Verification items for the finished model (mm, model axes). Face numbers are marked on the shaded views. A direction names the side the tool comes from. Give positions to 0.01 mm unless a question says otherwise; leave off trailing zeros. Order: outer loops, then holes, each group sorted by start corner. A loop starts at its lowest first (then second) coordinate and runs counter-clockwise, first axis right, second up.
from build123d import *

# Parameters (mm, degrees)
SKETCH1_W           = 21.9456
SKETCH1_H           = 10.033
SKETCH1_H_2         = 6.5151
BOSS_EXTRUDE1_DEPTH = 18.288
SKETCH2_W           = 15.748
SKETCH2_H           = 13.0048
BOSS_EXTRUDE2_DEPTH = 2.0066
SKETCH3_R           = 1.4605
CUT_EXTRUDE1_DEPTH  = 29.260148325


with BuildPart() as part:
    # Sketch1 → Boss-Extrude1 (new body)
    with BuildSketch(Plane(origin=(0, 0, 0), x_dir=(1, 0, 0), z_dir=(0, 1, 0))):
        with BuildLine():
            Line((-13.1826, -5.0165), (-10.9728, -5.0165))
            Line((-10.9728, -5.0165), (-10.9728, 5.0165))
            Line((-10.9728, 5.0165), (-13.1826, 5.0165))
            ThreePointArc((-13.1826, 5.0165), (-18.1991, 0), (-13.1826, -5.0165))
        make_face()
        Rectangle(SKETCH1_W, SKETCH1_H)
        with Locations((0, -8.27405)):
            Rectangle(SKETCH1_W, SKETCH1_H_2)
        with BuildLine():
            Line((10.9728, 5.0165), (10.9728, -5.0165))
            Line((10.9728, -5.0165), (13.1826, -5.0165))
            ThreePointArc((13.1826, -5.0165), (18.1991, 0), (13.1826, 5.0165))
            Line((13.1826, 5.0165), (10.9728, 5.0165))
        make_face()
        with Locations((0, 8.27405)):
            Rectangle(SKETCH1_W, SKETCH1_H_2)
    extrude(amount=BOSS_EXTRUDE1_DEPTH)

    # Sketch2 → Boss-Extrude2 (add)
    with BuildSketch(Plane(origin=(0, 18.288, 0), x_dir=(1, 0, 0), z_dir=(0, 1, 0))):
        with Locations((0, 1.8542)):
            Rectangle(SKETCH2_W, SKETCH2_H)
    extrude(amount=BOSS_EXTRUDE2_DEPTH)

    # Sketch3 → Cut-Extrude1 (cut, through all)
    with BuildSketch(Plane(origin=(0, 18.288, 0), x_dir=(1, 0, 0), z_dir=(0, 1, 0))):
        with Locations(Location((-13.1826, 0, 0), (0, 0, 270))):
            Circle(SKETCH3_R)
        with Locations(Location((13.1826, 0, 0), (0, 0, 270))):
            Circle(SKETCH3_R)
    extrude(amount=-CUT_EXTRUDE1_DEPTH, mode=Mode.SUBTRACT)


solid = part.part
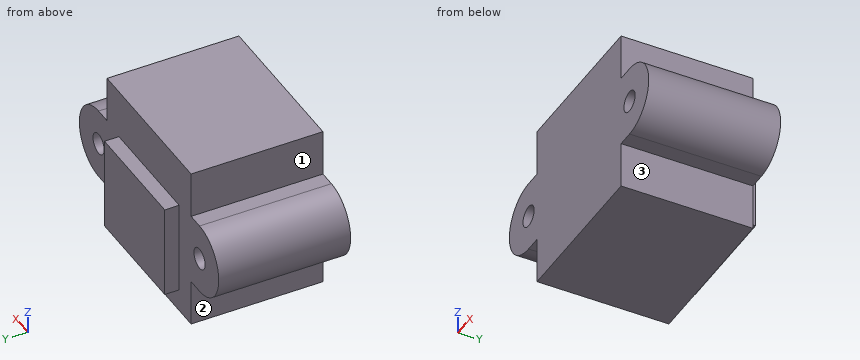
(1) Scan lines: line 1 (X direction, y = 11.25, z = 0); line 2 (X direction, y = 13.5, z = 1.25); line 3 (X direction, y = 7.75, z = -7.5). Record each from-to range of solid material in increasing order.
Solved:
line 1: x = -18.2 to -14.64, -11.72 to 11.72, 14.64 to 18.2
line 2: x = -18.04 to -13.94, -12.43 to 12.43, 13.94 to 18.04
line 3: x = -10.97 to 10.97
(2) Go/stop test with flat-tipped pins: pin 1 (1.5 mm diameter, centred on x = -13, y = 17, fed in from -Z); pin 2 (2 mm diameter, centred on x = 1, y = 19.5, fed in from +Z); pin 3 (2 mm diameter, centred on y = 13, z = -7.5, fed in from -X). Record where each tip stops, or that it passes through.
Solved:
pin 1: stops at z = -5.02
pin 2: stops at z = 4.65
pin 3: stops at x = -10.97
(3) Section check D-D, the plane z = -7.5. Enter the section's corners in (x, y).
Solved:
outline: (-10.97, 0) - (10.97, 0) - (10.97, 18.29) - (7.87, 18.29) - (7.87, 20.29) - (-7.87, 20.29) - (-7.87, 18.29) - (-10.97, 18.29) - close
(4) Set-up check for the marked faces 1, 2 and 3: record each of +Z, -Z, +X, -X, +Y, -Y from which the full face is reachable in a straight line by a thin tool's end or side.
Solved:
face 1: +Z, -X, +Y, -Y
face 2: -Z, -X, +Y, -Y
face 3: -Z, +X, +Y, -Y
(5) Section check B-B, the plane y = 1.5. Enter the section's corners in (x, z), then the cut area to 3 significant figures.
Solved:
outline: (-13.18, -5.02) - (-10.97, -5.02) - (-10.97, -11.53) - (10.97, -11.53) - (10.97, -5.02) - (13.18, -5.02) arc R5.02 ccw to (13.18, 5.02) - (10.97, 5.02) - (10.97, 11.53) - (-10.97, 11.53) - (-10.97, 5.02) - (-13.18, 5.02) arc R5.02 ccw to start; hole circle Ø2.92 at (-13.18, 0); hole circle Ø2.92 at (13.18, 0)
area: 616 mm2
(6) Section check C-C, the plane x = -2. Enter the section's corners in (y, z), then the cut area to 3 significant figures.
Solved:
outline: (0, -11.53) - (18.29, -11.53) - (18.29, -8.36) - (20.29, -8.36) - (20.29, 4.65) - (18.29, 4.65) - (18.29, 11.53) - (0, 11.53) - close
area: 448 mm2
(7) Section check A-A, the plane z = 0. Enter the section's corners in (x, y), then the cut area to 3 significant figures.
Solved:
outline: (-18.2, 0) - (-14.64, 0) - (-14.64, 18.29) - (-18.2, 18.29) - close; (-11.72, 0) - (11.72, 0) - (11.72, 18.29) - (7.87, 18.29) - (7.87, 20.29) - (-7.87, 20.29) - (-7.87, 18.29) - (-11.72, 18.29) - close; (14.64, 0) - (18.2, 0) - (18.2, 18.29) - (14.64, 18.29) - close
area: 590 mm2
